from build123d import *

# Parameters (mm, degrees)
Y_KSEKLIK_EKSTR_ZYON1_DEPTH = 2
IZIM2_W                     = 120
IZIM2_H                     = 2
Y_KSEKLIK_EKSTR_ZYON2_DEPTH = 38
RADYUS1_R                   = 10
RADYUS2_R                   = 5
IZIM3_R                     = 2
KES_EKSTR_ZYON1_DEPTH       = 2
RADYUS3_R                   = 3
IZIM4_R                     = 2
KES_EKSTR_ZYON2_DEPTH       = 101.498756211


with BuildPart() as part:
    # Çizim1 → Yükseklik-Ekstrüzyon1 (new body)
    with BuildSketch(Plane.XY):
        Polygon((-60, 20), (-35, 20), (-35, -20), (-60, -20), (-60, -35), (60, -35), (60, -20), (35, -20), (35, 20), (60, 20), (60, 35), (-60, 35), align=None)
    extrude(amount=Y_KSEKLIK_EKSTR_ZYON1_DEPTH)

    # Çizim2 → Yükseklik-Ekstrüzyon2 (add)
    with BuildSketch(Plane.XY.offset(2)):
        with Locations((0, 34)):
            Rectangle(IZIM2_W, IZIM2_H)
        with Locations((0, -34)):
            Rectangle(IZIM2_W, IZIM2_H)
    extrude(amount=Y_KSEKLIK_EKSTR_ZYON2_DEPTH)

    # Radyus1
    radyus1_edges = [part.edges().sort_by_distance(p)[0] for p in [
        (-60, 34, 40),
        (60, 34, 40),
        (60, -34, 40),
        (-60, -34, 40),
    ]]
    fillet(radyus1_edges, radius=RADYUS1_R)

    # Radyus2
    radyus2_edges = [part.edges().sort_by_distance(p)[0] for p in [
        (60, -20, 1),
        (60, 20, 1),
        (-60, -20, 1),
        (-60, 20, 1),
    ]]
    fillet(radyus2_edges, radius=RADYUS2_R)

    # Çizim3 → Kes-Ekstrüzyon1 (cut)
    with BuildSketch(Plane(origin=(0, 0, 0), x_dir=(-1, 0, 0), z_dir=(0, 0, -1))):
        with Locations((30, -25)):
            Circle(IZIM3_R)
        with Locations((40, -25)):
            Circle(IZIM3_R)
        with Locations((50, -25)):
            Circle(IZIM3_R)
        with Locations((20, -25)):
            Circle(IZIM3_R)
        with Locations((10, -25)):
            Circle(IZIM3_R)
        with Locations((0, -25)):
            Circle(IZIM3_R)
        with Locations((-10, -25)):
            Circle(IZIM3_R)
        with Locations((-20, -25)):
            Circle(IZIM3_R)
        with Locations((-30, -25)):
            Circle(IZIM3_R)
        with Locations((20, -15)):
            Circle(IZIM3_R)
        with Locations((10, -15)):
            Circle(IZIM3_R)
        with Locations((0, -15)):
            Circle(IZIM3_R)
        with Locations((-10, -15)):
            Circle(IZIM3_R)
        with Locations((-20, -15)):
            Circle(IZIM3_R)
        with Locations((-30, -15)):
            Circle(IZIM3_R)
        with Locations((20, -5)):
            Circle(IZIM3_R)
        with Locations((10, -5)):
            Circle(IZIM3_R)
        with Locations((0, -5)):
            Circle(IZIM3_R)
        with Locations((-10, -5)):
            Circle(IZIM3_R)
        with Locations((-20, -5)):
            Circle(IZIM3_R)
        with Locations((-30, -5)):
            Circle(IZIM3_R)
        with Locations((20, 5)):
            Circle(IZIM3_R)
        with Locations((10, 5)):
            Circle(IZIM3_R)
        with Locations((0, 5)):
            Circle(IZIM3_R)
        with Locations((-10, 5)):
            Circle(IZIM3_R)
        with Locations((-20, 5)):
            Circle(IZIM3_R)
        with Locations((-30, 5)):
            Circle(IZIM3_R)
        with Locations((20, 15)):
            Circle(IZIM3_R)
        with Locations((10, 15)):
            Circle(IZIM3_R)
        with Locations((0, 15)):
            Circle(IZIM3_R)
        with Locations((-10, 15)):
            Circle(IZIM3_R)
        with Locations((-20, 15)):
            Circle(IZIM3_R)
        with Locations((-30, 15)):
            Circle(IZIM3_R)
        with Locations((20, 25)):
            Circle(IZIM3_R)
        with Locations((10, 25)):
            Circle(IZIM3_R)
        with Locations((0, 25)):
            Circle(IZIM3_R)
        with Locations((-10, 25)):
            Circle(IZIM3_R)
        with Locations((-20, 25)):
            Circle(IZIM3_R)
        with Locations((-30, 25)):
            Circle(IZIM3_R)
        with Locations((30, -15)):
            Circle(IZIM3_R)
        with Locations((30, -5)):
            Circle(IZIM3_R)
        with Locations((30, 5)):
            Circle(IZIM3_R)
        with Locations((30, 15)):
            Circle(IZIM3_R)
        with Locations((30, 25)):
            Circle(IZIM3_R)
        with Locations((40, 25)):
            Circle(IZIM3_R)
        with Locations((50, 25)):
            Circle(IZIM3_R)
        with Locations((-40, 25)):
            Circle(IZIM3_R)
        with Locations((-50, 25)):
            Circle(IZIM3_R)
        with Locations((-40, -25)):
            Circle(IZIM3_R)
        with Locations((-50, -25)):
            Circle(IZIM3_R)
    extrude(amount=-KES_EKSTR_ZYON1_DEPTH, mode=Mode.SUBTRACT)

    # Radyus3
    radyus3_edges = [part.edges().sort_by_distance(p)[0] for p in [
        (0, 35, 0),
        (0, 33, 2),
        (0, -33, 2),
        (0, -35, 0),
    ]]
    fillet(radyus3_edges, radius=RADYUS3_R)

    # Çizim4 → Kes-Ekstrüzyon2 (cut, through all)
    with BuildSketch(Plane.XZ.offset(35)):
        with Locations(Location((0, 10, 0), (0, 0, 270))):
            Circle(IZIM4_R)
        with Locations(Location((20, 10, 0), (0, 0, 270))):
            Circle(IZIM4_R)
        with Locations(Location((40, 10, 0), (0, 0, 270))):
            Circle(IZIM4_R)
        with Locations(Location((20, 20, 0), (0, 0, 270))):
            Circle(IZIM4_R)
        with Locations(Location((40, 20, 0), (0, 0, 270))):
            Circle(IZIM4_R)
        with Locations(Location((20, 30, 0), (0, 0, 270))):
            Circle(IZIM4_R)
        with Locations(Location((40, 30, 0), (0, 0, 270))):
            Circle(IZIM4_R)
        with Locations(Location((0, 20, 0), (0, 0, 270))):
            Circle(IZIM4_R)
        with Locations(Location((0, 30, 0), (0, 0, 270))):
            Circle(IZIM4_R)
        with Locations(Location((-20, 10, 0), (0, 0, 270))):
            Circle(IZIM4_R)
        with Locations(Location((-40, 10, 0), (0, 0, 270))):
            Circle(IZIM4_R)
        with Locations(Location((-40, 20, 0), (0, 0, 270))):
            Circle(IZIM4_R)
        with Locations(Location((-40, 30, 0), (0, 0, 270))):
            Circle(IZIM4_R)
        with Locations(Location((-20, 20, 0), (0, 0, 270))):
            Circle(IZIM4_R)
        with Locations(Location((-20, 30, 0), (0, 0, 270))):
            Circle(IZIM4_R)
        with Locations(Location((30, 30, 0), (0, 0, 270))):
            Circle(IZIM4_R)
        with Locations(Location((-30, 30, 0), (0, 0, 270))):
            Circle(IZIM4_R)
        with Locations(Location((50, 10, 0), (0, 0, 270))):
            Circle(IZIM4_R)
        with Locations(Location((50, 20, 0), (0, 0, 270))):
            Circle(IZIM4_R)
        with Locations(Location((50, 30, 0), (0, 0, 270))):
            Circle(IZIM4_R)
        with Locations(Location((-50, 10, 0), (0, 0, 270))):
            Circle(IZIM4_R)
        with Locations(Location((-50, 20, 0), (0, 0, 270))):
            Circle(IZIM4_R)
        with Locations(Location((-50, 30, 0), (0, 0, 270))):
            Circle(IZIM4_R)
    extrude(amount=-KES_EKSTR_ZYON2_DEPTH, mode=Mode.SUBTRACT)


solid = part.part
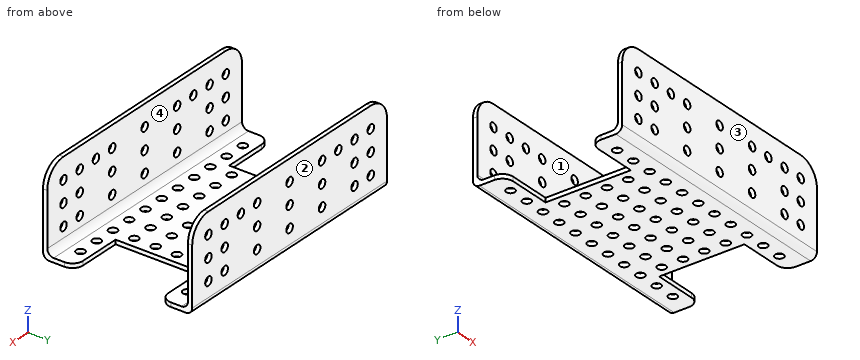
Could you check a few things on this model? Use its own coordinates, in mm. Face numbers are marked on the shaded views. Give positions to 0.01 mm unless a question says otherwise; leave off trailing zeros. Loops run counter-clockwise (first coordinate to the right, second up) from the corner with the lowest first, then second, coordinate; pieces in that order, holes last. Notation, with made-up numbers: (20, 55) -> (72, 55) arc R18 cw to (72, 80) -> close; hole circle Ø9 at (80.5, 89). An arc over 180 degrees is marked (long way). Answer as CSV lines item,"result". Start each with the question number.
(1) We'd pull the mould along Y, two halves only. Please class the marked faces 1, 2, 3 and 4: released by +Y, released by -Y, zero draft, split by the parting line, or undercut.
(2) If we section it at C-C on y = -8.5: Write out the boundary of the cut face in (x, z), then the cut area to 3 significant figures.
(3) If we section it at A-A on x = -15: Write out the boundary of the cut face in (y, z), then the cut area to 3 significant figures.
(4) If we section it at B-B on x = 10: Count the separate pieces of the cut face and the enclosed holes in it, then the cut area to 3 significant figures.
(5) I'm going to push flat-ended pins straight in: pin 1 Ø12 at (y, z) = (3, 9) entering from -X; pin 2 Ø1.6 at (x, z) = (-49.5, 1.5) entering from -Y; pin 3 Ø6.5 at (x, y) = (10, 5) entering from +Z; pin 4 Ø0.6 at (x, z) = (43.5, 1.5) entering from +Y. Where does each tip first touch, or does it pass through?
(6) I need wall thicknesses on probe 1 along Y at (x, z) = (50, 14); probe 2 along Z at (x, y) = (8, -24). Which ranges of each line are inside material? Lowest first, please.
Computed:
1,face 1,"undercut"
1,face 2,"released by +Y"
1,face 3,"released by -Y"
1,face 4,"undercut"
2,outline,"(-35, 0) -> (35, 0) -> (35, 2) -> (-35, 2) -> close"
2,area,"140 mm2"
3,outline,"(-35, 3) arc R3 ccw to (-32, 0) -> (32, 0) arc R3 ccw to (35, 3) -> (35, 40) -> (33, 40) -> (33, 5) arc R3 cw to (30, 2) -> (-30, 2) arc R3 cw to (-33, 5) -> (-33, 40) -> (-35, 40) -> close"
3,area,"292 mm2"
4,separate pieces,"7"
4,enclosed holes,"0"
4,area,"244 mm2"
5,pin 1,"passes through"
5,pin 2,"stops at y = -34.92"
5,pin 3,"stops at z = 2"
5,pin 4,"stops at y = 34.75"
6,probe 1,"y = -35 to -33, 33 to 35"
6,probe 2,"z = 0 to 2"
